Autodesk Inventor part; units mm, degrees
ref_plane "YZ Plane" through (0, 0, 0) normal (1, 0, 0) x (0, 1, 0)
ref_plane "XZ Plane" through (0, 0, 0) normal (0, 1, 0) x (-1, 0, 0)
ref_plane "XY Plane" through (0, 0, 0) normal (0, 0, 1) x (1, 0, 0)
sketch "Sketch1" plane through (0, 0, 0) normal (0, 1, 0) x (-1, 0, 0)
  line L0 (0, 0) -> (30, 0)
  line L1 (30, 0) -> (30, -10)
  line L2 (30, -10) -> (0, -10)
  line L3 (0, -10) -> (0, 0)
  dimension "d0" = 30
  dimension "d1" = 10
extrude "Extrusion1" add sketch "Sketch1" along normal blind 3
sketch "Sketch2" plane through (0, 3, 0) normal (0, 1, 0) x (1, 0, 0)
  line L0 (-30, 3) -> (-27, 3)
  line L1 (-27, 3) -> (-27, 4)
  line L2 (-27, 4) -> (-24, 4)
  line L3 (-24, 4) -> (-24, 5)
  line L4 (-24, 5) -> (-21, 5)
  line L5 (-21, 5) -> (-21, 6)
  line L6 (-21, 6) -> (-18, 6)
  line L7 (-18, 6) -> (-18, 7)
  line L8 (-18, 7) -> (-15, 7)
  line L9 (-15, 7) -> (-15, 8)
  line L10 (-15, 8) -> (-12, 8)
  line L11 (-12, 8) -> (-12, 9)
  line L12 (-12, 9) -> (-9, 9)
  line L13 (-9, 9) -> (-9, 10)
  line L14 (-9, 10) -> (-1.5529, 10)
  line L15 (-1.5529, 10) -> (-1.5529, 20)
  line L16 (-1.5529, 20) -> (-30, 20)
  line L17 (-30, 20) -> (-30, 3)
  line L18 (-30, 0) -> (0, 0)
  line L19 (-30, 10) -> (-30, 0)
  dimension "d4" = 3
  dimension "d5" = 3
  dimension "d6" = 3
  dimension "d7" = 3
  dimension "d8" = 3
  dimension "d9" = 3
  dimension "d10" = 1
  dimension "d11" = 1
  dimension "d12" = 1
  dimension "d13" = 1
  dimension "d14" = 1
  dimension "d15" = 1
  dimension "d16" = 3
  dimension "d17" = 1
  dimension "d18" = 3
  dimension "d19" = 10
  dimension "d20" = 28.4471
extrude "Extrusion2" cut sketch "Sketch2" against normal through all
properties part number "TRUC"
For this review, take the finished solid that the model builds, in its own axes (mm). A direction names the side the tool comes from. Coordinates: 2 decimals unless noted, no trailing zeros. Order: outer loops, then holes, each group sorted by start corner. A loop starts at its lowest first (then second) coordinate and runs counter-clockwise, first axis right, second up. Notation, with made-up numbers: (-3.5, -28) -> (50.5, -28) arc R28 cw to (50.5, -10) -> close; hole circle Ø7 at (75.5, -5.75). An arc over 180 degrees is marked (long way). Answer as CSV lines item,"result".
Q1. For faces 1 (the face through (-17, 2, -7)), 2 (the face through (-11, 0, -4)), list the 3-axis set-ups (+Z, -Z, +X, -X, +Y, -Y) from which the entire face can be reached by the end or side of a thin tool; tool diameter is ignored.
Model answer:
face 1,"-Z, -X, +Y, -Y"
face 2,"+Z, -Z, +X, -X, -Y"
Q2. Wall thickness on line 1 along X through (y, z) = (2.35, -3.25); line 2 along Z through (x, y) = (-12.25, 1.7); line 3 along Z through (x, y) = (-18.5, 1): over which ranges is each line inside the solid? List them lowest first. Write a range as [from, to].
Model answer:
line 1,"x = [-27, 0]"
line 2,"z = [-8, 0]"
line 3,"z = [-6, 0]"
Q3. We need section A-A (y = 0.8). State the section outline as (x, z) points.
Model answer:
outline,"(-30, -3) -> (-27, -3) -> (-27, -4) -> (-24, -4) -> (-24, -5) -> (-21, -5) -> (-21, -6) -> (-18, -6) -> (-18, -7) -> (-15, -7) -> (-15, -8) -> (-12, -8) -> (-12, -9) -> (-9, -9) -> (-9, -10) -> (0, -10) -> (0, 0) -> (-30, 0) -> close"
Q4. We need section B-B (z = -6.5). State the section outline as (x, y) points.
Model answer:
outline,"(-18, 0) -> (0, 0) -> (0, 3) -> (-18, 3) -> close"
Q5. We need section C-C (x = -17.5). State the section outline as (y, z) points, plus the area to 3 significant figures.
Model answer:
outline,"(0, -7) -> (3, -7) -> (3, 0) -> (0, 0) -> close"
area,"21.0 mm2"
Q6. Clearance check with flat-ended pins moving along their axes: pin 1 Ø0.5 at (y, z) = (1.5, -9.5) entering from -X; pin 2 Ø0.5 at (y, z) = (1, -4.5) entering from -X; pin 3 Ø0.8 at (y, z) = (1, -8.5) entering from -X. State where each tip first meets the part, or that it passes through.
Model answer:
pin 1,"stops at x = -9"
pin 2,"stops at x = -24"
pin 3,"stops at x = -12"
